CAD build for the part. Positions are in the model's coordinates, mm. Face numbers are marked on the shaded views. Coordinates: 2 decimals unless noted, no trailing zeros. Loops run counter-clockwise (first coordinate to the right, second up) from the corner with the lowest first, then second, coordinate; pieces in that order, holes last.
1) Saw through at A-A, the plane x = 0. Write the cut outline in (y, z).
2) Two-plate mould, pull along Z, no slides. Class the marked faces 1, 2, 3 and 4: +Z half, -Z half, draft (parallel to the pull), parting line (faces both ways), or undercut.
3) Pin check, flat tips, straight feed: pin 1 Ø5 at (y, z) = (0, 6.5) entering from +X; pin 2 Ø3 at (y, z) = (-2.5, 7) entering from +X; pin 3 Ø6 at (x, z) = (-3.5, 10) entering from -Y. Stop position of each tip, or through.
4) Wall check: line 1 along Z through (x, y) = (0.5, 4); line 2 along Y through (x, z) = (-3, 1); line 3 along X through (y, z) = (3.25, 4.25). Give the ranges that are in metal, low to high.
5) Saw through at B-B, the plane y = 0.25. Write the cut outline in (x, z), and give its area (3 significant figures).
6) Saw through at D-D, the plane z = 4.5. Write the cut outline in (x, y), and give its area (3 significant figures).
7) Saw through at C-C, the plane x = 4.5. Write the cut outline in (y, z).
```python
from build123d import *

# Parameters (mm, degrees)
F0_R     = 5
F1_DEPTH = 2.5
F2_R     = 4
F3_DEPTH = 3.6


with BuildPart() as f1:
    # F0 (on Top) → F1 (new body)
    with BuildSketch(Plane.XY):
        Circle(F0_R)
    extrude(amount=F1_DEPTH)

    # F2 (on face) → F3 (join)
    with BuildSketch(Plane.XY.offset(2.5)):
        Circle(F2_R)
    extrude(amount=F3_DEPTH)

    # F5: F1 across plane


with BuildPart() as f1_1:
    add(f1.part)
    add(f1.part.mirror(Plane.XY.offset(6.1)))


solid = f1_1.part
```
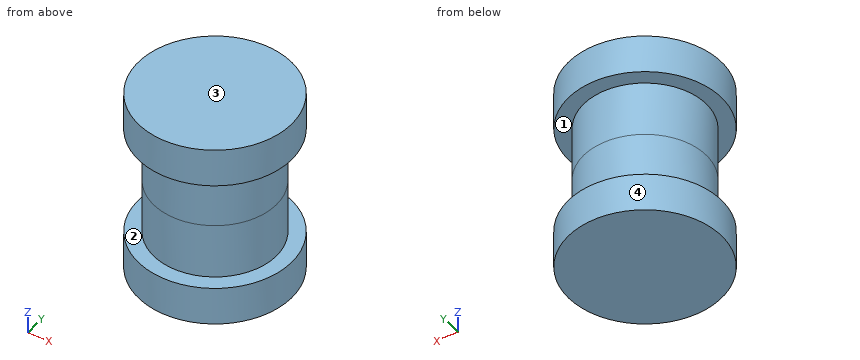
Data:
1. outline: (-5, 0) - (5, 0) - (5, 2.5) - (4, 2.5) - (4, 9.7) - (5, 9.7) - (5, 12.2) - (-5, 12.2) - (-5, 9.7) - (-4, 9.7) - (-4, 2.5) - (-5, 2.5) - close
2. face 1: undercut
2. face 2: undercut
2. face 3: +Z half
2. face 4: draft
3. pin 1: stops at x = 4
3. pin 2: stops at x = 3.87
3. pin 3: stops at y = -4.97
4. line 1: z = 0 to 2.5, 9.7 to 12.2
4. line 2: y = -4 to 4
4. line 3: x = -2.33 to 2.33
5. outline: (-4.99, 0) - (4.99, 0) - (4.99, 2.5) - (3.99, 2.5) - (3.99, 9.7) - (4.99, 9.7) - (4.99, 12.2) - (-4.99, 12.2) - (-4.99, 9.7) - (-3.99, 9.7) - (-3.99, 2.5) - (-4.99, 2.5) - close
5. area: 107 mm2
6. outline: circle Ø8 at (0, 0)
6. area: 50.3 mm2
7. outline: (-2.18, 0) - (2.18, 0) - (2.18, 2.5) - (-2.18, 2.5) - close; (-2.18, 9.7) - (2.18, 9.7) - (2.18, 12.2) - (-2.18, 12.2) - close
